Verification items for the finished model (mm, model axes). Give positions to 0.01 mm unless a question says otherwise; leave off trailing zeros. Order: outer loops, then holes, each group sorted by start corner. A loop starts at its lowest first (then second) coordinate and runs counter-clockwise, first axis right, second up. Notation, with made-up numbers: (62, 27) -> (82, 27) arc R8 cw to (82, 33) -> close; hole circle Ø1 at (57, 47.5). An arc over 180 degrees is marked (long way). Write each question's results on one line, items separated by ' | '. Start each with the question number.
1. Cross-section at B-B, the plane x = 213.5. Enter the section's corners in (y, z).
2. Mould release check, pull along X, two halves, no side actions. Record for faces 1 (the face through (-13.458, 12.878, -2.273)), 2 (the face through (96, 13, 38.1)), 3 (the face through (-70.772, 13, 0)): +X half, -X half, draft (parallel to the pull), parting line (faces both ways), or undercut.
3. Depth check by flat-ended pin: pin 1 Ø2 at (y, z) = (10.5, 15.5) entering from +X; pin 2 Ø1 at (y, z) = (13.5, 26) entering from +X; pin 3 Ø10 at (y, z) = (13.5, -22.5) entering from +X. Enter the tip coordinate at first touch or a pass-through.
4. Cross-section at A-A, the plane z = 0. Enter the section's corners in (x, y), then the cut area to 3 significant figures.
5. Material ranges on L1, parallel to X at y = 22, z = -1.5; L2, parallel to X at y = 14.25, z = -18.5; L3, parallel to X at y = 18.75, z = -5.5, recorded low to high. Write a range as from..to.
6. Cross-section at C-C, the plane y = 6.5. State how many separate pieces and enclosed holes the cut face has, then the cut area to 3 significant figures.
7. Cross-section at D-D, the plane z = 28. Enter the section's corners in (x, y).
from build123d import *

# Parameters (mm, degrees)
BOSS_EXTRUDE1_DEPTH = 25.4
CUT_EXTRUDE1_REACH  = 265.241
SKETCH5_R           = 6.35
SKETCH5_R_2         = 17.4625
CUT_EXTRUDE2_REACH  = 265.241
SKETCH6_R           = 1.5875


with BuildPart() as part:
    # Sketch4 → Boss-Extrude1 (new body)
    with BuildSketch(Plane(origin=(0, 0, 0), x_dir=(1, 0, 0), z_dir=(0, 1, 0))):
        with BuildLine():
            Line((233.827945205, -38.1), (-45.372054795, -38.1))
            ThreePointArc((-45.372054795, -38.1), (-63.332567037, -30.660512242), (-70.772054795, -12.7))
            Line((-70.772054795, -12.7), (-70.772054795, 12.7))
            ThreePointArc((-70.772054795, 12.7), (-63.332567037, 30.660512242), (-45.372054795, 38.1))
            Line((-45.372054795, 38.1), (233.827945205, 38.1))
            ThreePointArc((233.827945205, 38.1), (251.788457448, 30.660512242), (259.227945205, 12.7))
            Line((259.227945205, 12.7), (259.227945205, -12.7))
            ThreePointArc((259.227945205, -12.7), (251.788457448, -30.660512242), (233.827945205, -38.1))
        make_face()
    extrude(amount=BOSS_EXTRUDE1_DEPTH)

    # Sketch5 → Cut-Extrude1 (cut, up to next)
    with BuildSketch(Plane(origin=(0, 25.4, 0), x_dir=(1, 0, 0), z_dir=(0, 1, 0)), mode=Mode.PRIVATE) as cut_extrude1_sk1:
        with Locations(Location((94.227945205, 0, 0), (0, 0, 270))):
            Circle(SKETCH5_R)
    cut_extrude1_tool1 = extrude(cut_extrude1_sk1.sketch, amount=-CUT_EXTRUDE1_REACH, mode=Mode.PRIVATE) & part.part
    # Sketch5 → Cut-Extrude1 (cut, up to next)
    with BuildSketch(Plane(origin=(0, 25.4, 0), x_dir=(1, 0, 0), z_dir=(0, 1, 0)), mode=Mode.PRIVATE) as cut_extrude1_sk2:
        with Locations(Location((-30.772054795, 0, 0), (0, 0, 270))):
            Circle(SKETCH5_R_2)
    cut_extrude1_tool2 = extrude(cut_extrude1_sk2.sketch, amount=-CUT_EXTRUDE1_REACH, mode=Mode.PRIVATE) & part.part
    # Sketch5 → Cut-Extrude1 (cut, up to next)
    with BuildSketch(Plane(origin=(0, 25.4, 0), x_dir=(1, 0, 0), z_dir=(0, 1, 0)), mode=Mode.PRIVATE) as cut_extrude1_sk3:
        with Locations(Location((219.227945205, 0, 0), (0, 0, 270))):
            Circle(SKETCH5_R_2)
    cut_extrude1_tool3 = extrude(cut_extrude1_sk3.sketch, amount=-CUT_EXTRUDE1_REACH, mode=Mode.PRIVATE) & part.part
    add(cut_extrude1_tool1.solids().sort_by_distance((94.227945, 25.4, 0))[0], mode=Mode.SUBTRACT)
    add(cut_extrude1_tool2.solids().sort_by_distance((-30.772055, 25.4, 0))[0], mode=Mode.SUBTRACT)
    add(cut_extrude1_tool3.solids().sort_by_distance((219.227945, 25.4, 0))[0], mode=Mode.SUBTRACT)

    # Sketch6 → Cut-Extrude2 (cut, up to next)
    with BuildSketch(Plane.XZ, mode=Mode.PRIVATE) as cut_extrude2_sk1:
        with Locations(Location((201.709555727, 18.392009952, 0), (0, 0, 270))):
            Circle(SKETCH6_R)
    cut_extrude2_tool1 = extrude(cut_extrude2_sk1.sketch, amount=-CUT_EXTRUDE2_REACH, mode=Mode.PRIVATE) & part.part
    # Sketch6 → Cut-Extrude2 (cut, up to next)
    with BuildSketch(Plane.XZ, mode=Mode.PRIVATE) as cut_extrude2_sk2:
        with Locations(Location((237.619955157, 17.518389479, 0), (0, 0, 270))):
            Circle(SKETCH6_R)
    cut_extrude2_tool2 = extrude(cut_extrude2_sk2.sketch, amount=-CUT_EXTRUDE2_REACH, mode=Mode.PRIVATE) & part.part
    # Sketch6 → Cut-Extrude2 (cut, up to next)
    with BuildSketch(Plane.XZ, mode=Mode.PRIVATE) as cut_extrude2_sk3:
        with Locations(Location((236.746334684, -18.392009952, 0), (0, 0, 270))):
            Circle(SKETCH6_R)
    cut_extrude2_tool3 = extrude(cut_extrude2_sk3.sketch, amount=-CUT_EXTRUDE2_REACH, mode=Mode.PRIVATE) & part.part
    # Sketch6 → Cut-Extrude2 (cut, up to next)
    with BuildSketch(Plane.XZ, mode=Mode.PRIVATE) as cut_extrude2_sk4:
        with Locations(Location((200.835935254, -17.518389479, 0), (0, 0, 270))):
            Circle(SKETCH6_R)
    cut_extrude2_tool4 = extrude(cut_extrude2_sk4.sketch, amount=-CUT_EXTRUDE2_REACH, mode=Mode.PRIVATE) & part.part
    # Sketch6 → Cut-Extrude2 (cut, up to next)
    with BuildSketch(Plane.XZ, mode=Mode.PRIVATE) as cut_extrude2_sk5:
        with Locations(Location((-48.732567037, 17.960512242, 0), (0, 0, 270))):
            Circle(SKETCH6_R)
    cut_extrude2_tool5 = extrude(cut_extrude2_sk5.sketch, amount=-CUT_EXTRUDE2_REACH, mode=Mode.PRIVATE) & part.part
    # Sketch6 → Cut-Extrude2 (cut, up to next)
    with BuildSketch(Plane.XZ, mode=Mode.PRIVATE) as cut_extrude2_sk6:
        with Locations(Location((-12.811542552, 17.960512242, 0), (0, 0, 270))):
            Circle(SKETCH6_R)
    cut_extrude2_tool6 = extrude(cut_extrude2_sk6.sketch, amount=-CUT_EXTRUDE2_REACH, mode=Mode.PRIVATE) & part.part
    # Sketch6 → Cut-Extrude2 (cut, up to next)
    with BuildSketch(Plane.XZ, mode=Mode.PRIVATE) as cut_extrude2_sk7:
        with Locations(Location((-12.811542552, -17.960512242, 0), (0, 0, 270))):
            Circle(SKETCH6_R)
    cut_extrude2_tool7 = extrude(cut_extrude2_sk7.sketch, amount=-CUT_EXTRUDE2_REACH, mode=Mode.PRIVATE) & part.part
    # Sketch6 → Cut-Extrude2 (cut, up to next)
    with BuildSketch(Plane.XZ, mode=Mode.PRIVATE) as cut_extrude2_sk8:
        with Locations(Location((-48.732567037, -17.960512242, 0), (0, 0, 270))):
            Circle(SKETCH6_R)
    cut_extrude2_tool8 = extrude(cut_extrude2_sk8.sketch, amount=-CUT_EXTRUDE2_REACH, mode=Mode.PRIVATE) & part.part
    add(cut_extrude2_tool1.solids().sort_by_distance((201.709556, 0, 18.39201))[0], mode=Mode.SUBTRACT)
    add(cut_extrude2_tool2.solids().sort_by_distance((237.619955, 0, 17.518389))[0], mode=Mode.SUBTRACT)
    add(cut_extrude2_tool3.solids().sort_by_distance((236.746335, 0, -18.39201))[0], mode=Mode.SUBTRACT)
    add(cut_extrude2_tool4.solids().sort_by_distance((200.835935, 0, -17.518389))[0], mode=Mode.SUBTRACT)
    add(cut_extrude2_tool5.solids().sort_by_distance((-48.732567, 0, 17.960512))[0], mode=Mode.SUBTRACT)
    add(cut_extrude2_tool6.solids().sort_by_distance((-12.811543, 0, 17.960512))[0], mode=Mode.SUBTRACT)
    add(cut_extrude2_tool7.solids().sort_by_distance((-12.811543, 0, -17.960512))[0], mode=Mode.SUBTRACT)
    add(cut_extrude2_tool8.solids().sort_by_distance((-48.732567, 0, -17.960512))[0], mode=Mode.SUBTRACT)


solid = part.part
Results below:
1) outline: (0, -38.1) -> (25.4, -38.1) -> (25.4, -16.5) -> (0, -16.5) -> close; (0, 16.5) -> (25.4, 16.5) -> (25.4, 38.1) -> (0, 38.1) -> close
2) face 1: undercut | face 2: draft | face 3: -X half
3) pin 1: stops at x = 259.16 | pin 2: stops at x = 255.77 | pin 3: stops at x = 258.77
4) outline: (-70.77, 0) -> (-48.23, 0) -> (-48.23, 25.4) -> (-70.77, 25.4) -> close; (-13.31, 0) -> (87.88, 0) -> (87.88, 25.4) -> (-13.31, 25.4) -> close; (100.58, 0) -> (201.77, 0) -> (201.77, 25.4) -> (100.58, 25.4) -> close; (236.69, 0) -> (259.23, 0) -> (259.23, 25.4) -> (236.69, 25.4) -> close | area: 6,290 mm²
5) L1: x = -70.77..-48.17, -13.37..88.06, 100.4..201.83, 236.63..259.23 | L2: x = -70.1..-50.23, -47.24..-14.3, -11.32..199.59, 202.08..235.16, 238.33..258.56 | L3: x = -70.77..-47.35, -14.2..91.05, 97.4..202.65, 235.8..259.23
6) separate pieces: 1 | enclosed holes: 11 | area: 22,500 mm²
7) outline: (-65.65, 0) -> (254.1, 0) -> (254.1, 25.4) -> (-65.65, 25.4) -> close
